```python
from build123d import *

# Parameters (mm, degrees)
SKETCH1_R                = 2.38125
BOSS_EXTRUDE1_DEPTH      = 38.1
FILLET1_R                = 6.35
SKETCH3_W                = 38.1
SKETCH3_H                = 6.35
BOSS_EXTRUDE2_DEPTH      = 12.7
SKETCH2_W                = 7.62
SKETCH2_H                = 8.89
CUT_EXTRUDE7_DEPTH       = 66.019560197
BOSS_EXTRUDE5_DEPTH      = 22.225
BOSS_EXTRUDE5_DEPTH_BACK = 9.525
SKETCH10_W               = 7.62
SKETCH10_H               = 8.89
CUT_EXTRUDE1_DEPTH       = 62.376176621
CUT_EXTRUDE1_DEPTH_BACK  = 62.376176621
SKETCH5_R                = 1.905
SKETCH6_W                = 8.89
SKETCH6_H                = 8.89
BOSS_EXTRUDE4_DEPTH      = 3.175
CUT_EXTRUDE2_DEPTH       = 71.485759779
CUT_EXTRUDE2_DEPTH_BACK  = 71.485759779
SKETCH7_R                = 2.0828
CUT_EXTRUDE8_DEPTH       = 13.335
SKETCH11_W               = 7.62
SKETCH11_H               = 8.89
CUT_EXTRUDE9_DEPTH       = 68.896996404
SKETCH12_W               = 8.89
SKETCH12_H               = 8.89
CUT_EXTRUDE10_DEPTH      = 3.175
CUT_EXTRUDE11_DEPTH      = 58.406346519


with BuildPart() as part:
    # Sketch1 → Boss-Extrude1 (new body)
    with BuildSketch(Plane.XY):
        with BuildLine():
            Line((-37.385625, -8.255), (-37.385625, -3.175))
            Line((-37.385625, -3.175), (-37.385625, 3.175))
            Line((-37.385625, 3.175), (37.385625, 3.175))
            Line((37.385625, 3.175), (37.385625, -3.175))
            Line((37.385625, -3.175), (-27.543125, -3.175))
            Line((-27.543125, -3.175), (-27.543125, -8.255))
            ThreePointArc((-27.543125, -8.255), (-32.464375, -13.17625), (-37.385625, -8.255))
        make_face()
        with Locations(Location((-32.464375, -8.255, 0), (0, 0, 180))):
            Circle(SKETCH1_R, mode=Mode.SUBTRACT)
    extrude(amount=BOSS_EXTRUDE1_DEPTH)

    # Fillet1
    fillet1_edges = [part.edges().sort_by_distance(p)[0] for p in [
        (-37.385625, 3.175, 19.05),
    ]]
    fillet(fillet1_edges, radius=FILLET1_R)

    # Sketch3 → Boss-Extrude2 (add)
    with BuildSketch(Plane(origin=(37.385625, 0, 0), x_dir=(0, 0, -1), z_dir=(1, 0, 0))):
        with Locations((-19.05, 0)):
            Rectangle(SKETCH3_W, SKETCH3_H)
    extrude(amount=BOSS_EXTRUDE2_DEPTH)

    # Sketch2 → Cut-Extrude7 (cut, through all)
    with BuildSketch(Plane(origin=(0, 3.175, 0), x_dir=(1, 0, 0), z_dir=(0, 1, 0))):
        with Locations((17.541875, -20.32)):
            Rectangle(SKETCH2_W, SKETCH2_H)
    extrude(amount=-CUT_EXTRUDE7_DEPTH, mode=Mode.SUBTRACT)

    # Sketch10 → Boss-Extrude5 (add, two sides: drawn at the far end of the back side and taken through both)
    with BuildSketch(Plane(origin=(0, 3.175, 0), x_dir=(1, 0, 0), z_dir=(0, 1, 0)).offset(-BOSS_EXTRUDE5_DEPTH_BACK)):
        with Locations((17.541875, -20.32)):
            Rectangle(SKETCH10_W, SKETCH10_H)
    extrude(amount=BOSS_EXTRUDE5_DEPTH + BOSS_EXTRUDE5_DEPTH_BACK)

    # Sketch5 → Cut-Extrude1 (cut, two sides: drawn at the far end of the back side and taken through both)
    with BuildSketch(Plane.XY.offset(24.765).offset(-CUT_EXTRUDE1_DEPTH_BACK)):
        with Locations((17.541875, 5.715)):
            Circle(SKETCH5_R)
        with Locations((17.541875, 23.1775)):
            Circle(SKETCH5_R)
    extrude(amount=CUT_EXTRUDE1_DEPTH + CUT_EXTRUDE1_DEPTH_BACK, mode=Mode.SUBTRACT)

    # Sketch6 → Boss-Extrude4 (add)
    with BuildSketch(Plane(origin=(0, -3.175, 0), x_dir=(1, 0, 0), z_dir=(0, 1, 0))):
        with Locations((9.286875, -20.32)):
            Rectangle(SKETCH6_W, SKETCH6_H)
        with Locations((25.796875, -20.32)):
            Rectangle(SKETCH6_W, SKETCH6_H)
    extrude(amount=-BOSS_EXTRUDE4_DEPTH)

    # Sketch7 → Cut-Extrude2 (cut, two sides: drawn at the far end of the back side and taken through both)
    with BuildSketch(Plane(origin=(0, -6.35, 0), x_dir=(-1, 0, 0), z_dir=(0, -1, 0)).offset(-CUT_EXTRUDE2_DEPTH_BACK)):
        with Locations(Location((-9.286875, -20.32, 0), (0, 0, 90))):
            Circle(SKETCH7_R)
        with Locations(Location((-25.796875, -20.32, 0), (0, 0, 90))):
            Circle(SKETCH7_R)
    extrude(amount=CUT_EXTRUDE2_DEPTH + CUT_EXTRUDE2_DEPTH_BACK, mode=Mode.SUBTRACT)

    # Sketch9 → Cut-Extrude8 (cut)
    with BuildSketch(Plane.XY.offset(38.1)):
        with BuildLine():
            Line((50.085625, 3.175), (50.085625, -3.175))
            Line((50.085625, -3.175), (-27.543125, -3.175))
            Line((-27.543125, -3.175), (-27.543125, -8.255))
            ThreePointArc((-27.543125, -8.255), (-32.464375, -13.17625), (-37.385625, -8.255))
            Line((-37.385625, -8.255), (-37.385625, -3.175))
            ThreePointArc((-37.385625, -3.175), (-35.525753061, 1.315128061), (-31.035625, 3.175))
            Line((-31.035625, 3.175), (50.085625, 3.175))
        make_face()
    extrude(amount=-CUT_EXTRUDE8_DEPTH, mode=Mode.SUBTRACT)

    # Sketch11 → Cut-Extrude9 (cut, through all)
    with BuildSketch(Plane(origin=(0, 25.4, 0), x_dir=(1, 0, 0), z_dir=(0, 1, 0))):
        with Locations((17.541875, -20.32)):
            Rectangle(SKETCH11_W, SKETCH11_H)
    extrude(amount=-CUT_EXTRUDE9_DEPTH, mode=Mode.SUBTRACT)

    # Sketch12 → Cut-Extrude10 (cut)
    with BuildSketch(Plane.XZ.offset(6.35)):
        with Locations((9.286875, 20.32)):
            Rectangle(SKETCH12_W, SKETCH12_H)
        with Locations((25.796875, 20.32)):
            Rectangle(SKETCH12_W, SKETCH12_H)
    extrude(amount=-CUT_EXTRUDE10_DEPTH, mode=Mode.SUBTRACT)

    # Sketch13 → Cut-Extrude11 (cut, through all)
    with BuildSketch(Plane.XY.offset(24.765)):
        with BuildLine():
            Line((34.051875, 3.175), (50.085625, 3.175))
            Line((50.085625, 3.175), (50.085625, -3.175))
            Line((50.085625, -3.175), (34.051875, -3.175))
            ThreePointArc((34.051875, -3.175), (37.226875, 0), (34.051875, 3.175))
        make_face()
    extrude(amount=-CUT_EXTRUDE11_DEPTH, mode=Mode.SUBTRACT)


solid = part.part
```
Build history of the part. All positions in model axes, mm. A direction names the side the tool comes from. Give positions to 0.01 mm unless a question says otherwise; leave off trailing zeros. Order: outer loops, then holes, each group sorted by start corner. A loop starts at its lowest first (then second) coordinate and runs counter-clockwise, first axis right, second up. Notation, with made-up numbers: M 74,-12.5 L 91,-12.5 A10 ccw 91,2.5 Z; hole C -39,57 d8. An arc over 180 degrees is marked long. Write item = value, one per line. Start each with the question number.
(1) Probe L1, parallel to X at y = 1, z = 20.32; L2, parallel to Y at x = 3, z = 11.25 (3 decimals); L3, parallel to X at y = 1.75, z = 20.32. List the from-to ranges inside material, lowest first. Write a range as [from, to].
(2) Two-plate mould, pull along X, no slides. Class faces 1 (the flat face through (13.732, 0, 20)), 2 (the flat face through (-37.386, -6, 12)), 3 (the flat face through (1, 3.175, 13)), 4 (the cylindrical face through (8.489, 0.044, 18.396)): released by +X, released by -X, zero draft, split by the parting line, or undercut.
(3) Pin check, flat tips, straight feed: pin 1 Ø2.5 at (y, z) = (-4.5, 10) entering from +X; pin 2 Ø7 at (y, z) = (0, 20) entering from -X; pin 3 Ø7.5 at (x, z) = (18, 7.5) entering from -Y (3 decimals); pin 4 Ø1.9 at (x, y) = (17.5, -1) entering from +Z (3 decimals). Stop position of each tip, or through.
(4) Slice it at D-D on y = 0.25. Write the cut outline in (x, z) (3 decimals), plus the area to 3 significant figures.
(5) Slice it at C-C on x = 25. Write the cut outline in (y, z) (3 decimals), plus the area to 3 significant figures.
(6) Slice it at A-A on z = 20.32. State how many separate pieces and enclosed holes the cut face has, plus the area to 3 significant figures.
(7) Which spindle directions (+Z, -Z, +X, -X, +Y, -Y) get a long thin tool onto all of the face, cutting with end or side? Do faces 5 (the flat face through (3, -3.175, 13)), 6 (the flat face through (17, 0, 15.875)), 7 (the flat face through (-9, -1, 0)). Say none if no direction does.
Responses:
q1.L1 = [-35.82, 7.2], [11.37, 13.73], [21.35, 23.71], [27.88, 37.07]
q1.L2 = [-3.175, 3.175]
q1.L3 = [-35.04, 7.2], [11.37, 13.73], [21.35, 23.71], [27.88, 36.7]
q2.face_1 = undercut
q2.face_2 = released by -X
q2.face_3 = zero draft
q2.face_4 = undercut
q3.pin_1 = -27.54
q3.pin_2 = -37.39
q3.pin_3 = -3.175
q3.pin_4 = 15.875
q4.outline = M -36.383,0 L 37.217,0 L 37.217,24.765 L 21.352,24.765 L 21.352,15.875 L 13.732,15.875 L 13.732,24.765 L -36.383,24.765 Z; hole C 9.287,20.32 d4.166; hole C 25.797,20.32 d4.166
q4.area = 1,730 mm2
q5.outline = M -3.175,0 L 3.175,0 L 3.175,18.396 L -3.175,18.396 Z; M -3.175,22.244 L 3.175,22.244 L 3.175,24.765 L -3.175,24.765 Z
q5.area = 133 mm2
q6.separate_pieces = 4
q6.enclosed_holes = 1
q6.area = 430 mm2
q7.face_5 = +Z, -Z, +X, -Y
q7.face_6 = +Z, +Y, -Y
q7.face_7 = -Z, +X, -X, +Y, -Y
